```python
from build123d import *

# Parameters (mm, degrees)
F1_DEPTH = 12.7


with BuildPart() as f1:
    # F0 (on Right) → F1 (new body, symmetric)
    with BuildSketch(Plane.YZ):
        Polygon((-114.3, 136.525), (-215.9, 136.525), (-215.9, -136.525), (215.9, -136.525), (215.9, 136.525), (114.3, 136.525), (0, 85.725), align=None)
    extrude(amount=F1_DEPTH, both=True)


solid = f1.part
```
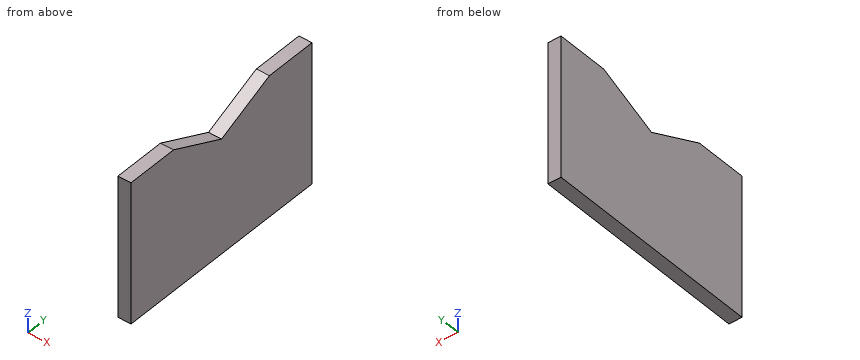
Could you check a few things on this model? Use its own coordinates, in mm. Coordinates: 2 decimals unless noted, no trailing zeros. Write each loop counter-clockwise with the first axis right and the second up, starting at its lowest first coordinate (ties: lowest second). Pieces come first, ordered by that corner, then holes. Notation, with made-up numbers: M 24.25,20 L 69.25,20 A25 cw 69.25,58 Z; hole C 82,-7.5 d3. An arc over 180 degrees is marked long. Answer as CSV lines item,"result". Start each with the question number.
1) I want a section at D-D, the plane y = -41.5. Please give me the cut outline in (x, z) (3 decimals).
2) For P1, Ø1, axis at x = 2, y = -47, coming from the +Z side; P2, Ø3, axis at x = 8.5, y = -23.5, coming from the +Z side, each with a flat end and sliding along its axis, tell me the tip position at first contact or that it passes through.
3) Please list where these lines run through material, in increasing order: line 1 (Y direction, x = 4.75, z = 95); line 2 (Y direction, x = 11.75, z = 112.5); line 3 (Z direction, x = -3.75, y = 32) (3 decimals). Write a range as from..to.
4) I want a section at C-C, the plane y = 64.5. Please give me the cut outline in (x, z) (3 decimals).
5) I want a section at B-B, the plane z = 97. Please give me the cut outline in (x, y), and give its area (3 significant figures).
6) I want a section at A-A, the plane x = 3.25. Please give me the cut outline in (y, z) (3 decimals).
Data:
1,outline,"M -12.7,-136.525 L 12.7,-136.525 L 12.7,104.169 L -12.7,104.169 Z"
2,P1,"stops at z = 106.84"
2,P2,"stops at z = 96.84"
3,line 1,"y = -215.9..-20.87, 20.87..215.9"
3,line 2,"y = -215.9..-60.24, 60.24..215.9"
3,line 3,"z = -136.525..99.947"
4,outline,"M -12.7,-136.525 L 12.7,-136.525 L 12.7,114.392 L -12.7,114.392 Z"
5,outline,"M -12.7,-215.9 L 12.7,-215.9 L 12.7,-25.37 L -12.7,-25.37 Z; M -12.7,25.37 L 12.7,25.37 L 12.7,215.9 L -12.7,215.9 Z"
5,area,"9,680 mm^2"
6,outline,"M -215.9,-136.525 L 215.9,-136.525 L 215.9,136.525 L 114.3,136.525 L 0,85.725 L -114.3,136.525 L -215.9,136.525 Z"
